Part model, mm, in its own coordinate system. A direction names the side the tool comes from. Round coordinates to 2 decimals unless told otherwise and drop trailing zeros. Order: outer loops, then holes, each group sorted by start corner. A loop starts at its lowest first (then second) coordinate and runs counter-clockwise, first axis right, second up. Notation, with made-up numbers: (4.25, 59) - (36.25, 59) arc R21 ccw to (36.25, 83) - close; hole circle Ø9 at (33, -1). An arc over 180 degrees is marked (long way). Answer as a JSON object with one key per item and string values.
```python
from build123d import *

# Parameters (mm, degrees)
SKETCH_1_W      = 43
SKETCH_1_H      = 40
SKETCH_1_R      = 2.15
EXTRUDE_1_DEPTH = 2
SKETCH_3_R      = 1.6
EXTRUDE_2_DEPTH = 2


with BuildPart() as part:
    # 草图1 → 凸台-拉伸1 (new body)
    with BuildSketch(Plane(origin=(0, 0, 0), x_dir=(1, 0, 0), z_dir=(0, 1, 0))):
        Rectangle(SKETCH_1_W, SKETCH_1_H)
        with Locations(Location((13, 15, 0), (0, 0, 270))):
            Circle(SKETCH_1_R, mode=Mode.SUBTRACT)
        with Locations(Location((13, -15, 0), (0, 0, 90))):
            Circle(SKETCH_1_R, mode=Mode.SUBTRACT)
        with Locations(Location((-11, 15, 0), (0, 0, 90))):
            Circle(SKETCH_1_R, mode=Mode.SUBTRACT)
        with Locations(Location((-11, -15, 0), (0, 0, 270))):
            Circle(SKETCH_1_R, mode=Mode.SUBTRACT)
    extrude(amount=EXTRUDE_1_DEPTH)

    # 草图3 → 凸台-拉伸2 (add)
    with BuildSketch(Plane.ZY.offset(21.5)):
        with BuildLine():
            Line((-20, 0), (-20, 26))
            ThreePointArc((-20, 26), (0, 46), (20, 26))
            Line((20, 26), (20, 0))
            Line((20, 0), (-20, 0))
        make_face()
        with Locations((-15.5, 26)):
            Circle(SKETCH_3_R, mode=Mode.SUBTRACT)
        with Locations((-7.75, 39.423393759)):
            Circle(SKETCH_3_R, mode=Mode.SUBTRACT)
        with Locations((7.75, 39.423393759)):
            Circle(SKETCH_3_R, mode=Mode.SUBTRACT)
        with Locations((15.5, 26)):
            Circle(SKETCH_3_R, mode=Mode.SUBTRACT)
        with Locations((7.75, 12.576606241)):
            Circle(SKETCH_3_R, mode=Mode.SUBTRACT)
        with Locations((-7.75, 12.576606241)):
            Circle(SKETCH_3_R, mode=Mode.SUBTRACT)
        with BuildLine():
            Line((-6, 18), (-6, 34))
            ThreePointArc((-6, 34), (0, 40), (6, 34))
            Line((6, 34), (6, 18))
            ThreePointArc((6, 18), (0, 12), (-6, 18))
        make_face(mode=Mode.SUBTRACT)
    extrude(amount=-EXTRUDE_2_DEPTH)


solid = part.part
```
Item 1: Tool access for faces 1 (the flat face through (-21, 26, -6)), 2 (the cylindrical face through (-10.35, 0.99, 17.05)), 3 (the flat face through (1, 2, 0)): list every direction of +Z, -Z, +X, -X, +Y, -Y with a clear straight run to the whole face (end or side of a thin tool).
Taken from the geometry:
{"face 1": "+X, -X", "face 2": "+Y, -Y", "face 3": "+Z, -Z, +X, +Y"}
Item 2: Cut at B-B (y = 31). Write the cut outline in (x, z), plus the area to 3 significant figures.
Taken from the geometry:
{"outline": "(-21.5, -19.36) - (-19.5, -19.36) - (-19.5, -6) - (-21.5, -6) - close; (-21.5, 6) - (-19.5, 6) - (-19.5, 19.36) - (-21.5, 19.36) - close", "area": "53.5 mm2"}
Item 3: Cut at A-A (z = 0). Write the cut outline in (x, y).
Taken from the geometry:
{"outline": "(-21.5, 0) - (21.5, 0) - (21.5, 2) - (-19.5, 2) - (-19.5, 12) - (-21.5, 12) - close; (-21.5, 40) - (-19.5, 40) - (-19.5, 46) - (-21.5, 46) - close"}
Item 4: Drop flat-ended pins along their axis: P1, Ø5, axis at y = 31, z = -7, coming from the +X side; P2, Ø12, axis at x = -1, z = 1, coming from the +Y side; P3, Ø3.5, axis at y = 12.58, z = -7.75, coming from the -X side. Give the stop position or say it passes through.
Taken from the geometry:
{"P1": "x = -19.5", "P2": "y = 2", "P3": "x = -21.5"}
Item 5: Two-plate mould, pull along Z, no slides. Class faces 4 (the cylindrical face through (-21, 40, 0)), 5 (the flat face through (-6, 1, -20)), 6 (the flat face through (-6, 1, 20)): pulls with the +Z half, pulls with the -Z half, needs draft (parallel to the pull), parting line crosses it, or undercut.
Taken from the geometry:
{"face 4": "undercut", "face 5": "pulls with the -Z half", "face 6": "pulls with the +Z half"}
Item 6: Cut at C-C (x = 11.5). Write the cut outline in (y, z).
Taken from the geometry:
{"outline": "(0, -20) - (2, -20) - (2, -16.54) - (0, -16.54) - close; (0, -13.46) - (2, -13.46) - (2, 13.46) - (0, 13.46) - close; (0, 16.54) - (2, 16.54) - (2, 20) - (0, 20) - close"}
Item 7: Probe L1, parallel to Y at x = -20, z = 7 (3 decimals); L2, parallel to Y at x = -14, z = 9.5; L3, parallel to X at y = 41.5, z = 0. List the from-to ranges inside material, lowest first. Write a range as from..to.
Taken from the geometry:
{"L1": "0..11.163, 13.99..38.01, 40.837..44.735", "L2": "0..2", "L3": "-21.5..-19.5"}
Item 8: Cut at D-D (z = 15). Write the cut outline in (x, y).
Taken from the geometry:
{"outline": "(-21.5, 0) - (-13.15, 0) - (-13.15, 2) - (-19.5, 2) - (-19.5, 24.48) - (-21.5, 24.48) - close; (-21.5, 27.52) - (-19.5, 27.52) - (-19.5, 39.23) - (-21.5, 39.23) - close; (-8.85, 0) - (10.85, 0) - (10.85, 2) - (-8.85, 2) - close; (15.15, 0) - (21.5, 0) - (21.5, 2) - (15.15, 2) - close"}
